Autodesk Inventor part; units mm, degrees
ref_plane "YZ Plane" through (0, 0, 0) normal (1, 0, 0) x (0, 1, 0)
ref_plane "XZ Plane" through (0, 0, 0) normal (0, 1, 0) x (-1, 0, 0)
ref_plane "XY Plane" through (0, 0, 0) normal (0, 0, 1) x (1, 0, 0)
sketch "Sketch1" plane through (0, 0, 0) normal (0, 0, 1) x (1, 0, 0)
  line L0 (21, -21) -> (-21, -21)
  line L1 (-21, -21) -> (-21, 21)
  line L2 (-21, 21) -> (21, 21)
  line L3 (21, 21) -> (21, -21)
  line L4 (21, -21) -> (-21, 21) construction
  line L5 (-21, -21) -> (21, 21) construction
  point P0 (0, 0)
  dimension "d0" = 42
extrude "Extrusion1" add sketch "Sketch1" along normal blind 48
sketch "Sketch2" plane through (0, 0, 48) normal (0, 0, 1) x (1, 0, 0)
  point P0 (0, 0)
  point P1 (-15.5, 15.5)
  point P2 (-15.5, -15.5)
  point P3 (15.5, -15.5)
  point P4 (15.5, 15.5)
  dimension "d3" = 31
  dimension "d4" = 31
  dimension "d5" = 15.5
  dimension "d6" = 15.5
hole "Hole1" at (-15.5, 15.5, 48) at (-15.5, -15.5, 48) at (15.5, -15.5, 48) at (15.5, 15.5, 48) direction (0, 0, -1) diameter 3 depth 8 tip angle 118
chamfer "Chamfer1" distance 3.5 angle 45 4 edges at (21, 21, 24) (21, -21, 24) (-21, 21, 24) (-21, -21, 24)
sketch "Sketch3" plane through (0, 0, 48) normal (0, 0, 1) x (1, 0, 0)
  circle A0 centre (0, 0) radius 11
  dimension "d17" = 22
extrude "Extrusion2" add sketch "Sketch3" along normal blind 2
sketch "Sketch4" plane through (0, 0, 50) normal (0, 0, 1) x (1, 0, 0)
  circle A0 centre (0, 0) radius 11
  circle A1 centre (0, 0) radius 2.5
  dimension "d20" = 5
extrude "Extrusion3" add sketch "Sketch4" along normal blind 25 contours A1
properties part number "Motor_XY" material "Steel, Alloy"
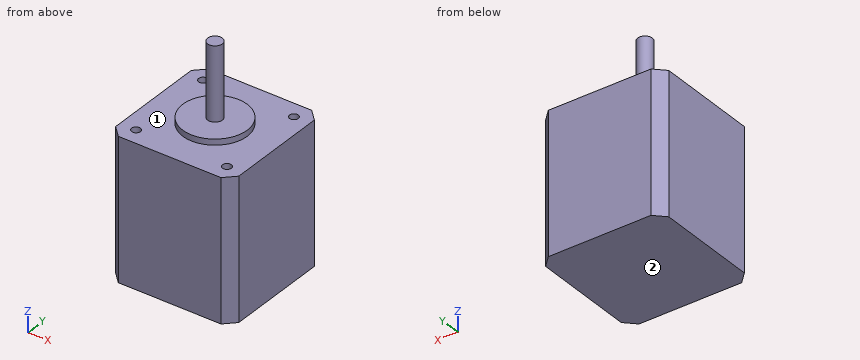
For this review, take the finished solid that the model builds, in its own axes (mm). Face numbers are marked on the shaded views. A direction names the side the tool comes from. Give positions to 0.01 mm unless a question says otherwise; leave off trailing zeros. Loops run counter-clockwise (first coordinate to the right, second up) from the corner with the lowest first, then second, coordinate; pieces in that order, holes last. Notation, with made-up numbers: M 55,62.25 L 108,62.25 A12 ccw 108,83.25 Z; hole C -15,13.25 d5. An arc over 180 degrees is marked long. Put each result on its own line as item: value. Start each with the question number.
(1) For pin 1 (2 mm diameter, centred on x = 7, y = -4, fed in from +Z); pin 2 (3 mm diameter, centred on y = 0.5, z = 56.5, fed in from -X); pin 3 (2.5 mm diameter, centred on x = 15.5, y = -15.5, fed in from +Z), all flat-tipped, find the tip position at first contact; note any pin that passes through.
(2) Wall thickness on L1, parallel to Y at x = 15.5, z = 45.25; L2, parallel to Y at x = -15, z = 46: over which ranges is each line inside the solid? List them lowest first.
(3) Machinability: for the marked faces 1 and 2, which of the approach directions +Z, -Z, +X, -X, +Y, -Y give a long, thin tool a straight path to every point of the face, cutting with its end or side? Answer none if there is none.
(4) Add section D-D, the plane y = 12.5. Write out the cut boundary in (x, z), then the cut area to 3 significant figures.
(5) Add section B-B, the plane x = 6. Write out the cut boundary in (y, z), then the cut area to 3 significant figures.
(6) Add section A-A, the plane y = 0. Write out the cut boundary in (x, z), then the cut area to 4 significant figures.
(7) Add section C-C, the plane z = 62.5. Write out the cut boundary in (x, y).
Result:
1. pin 1: stops at z = 50
1. pin 2: stops at x = -2.5
1. pin 3: stops at z = 39.85
2. L1: y = -21 to -17, -14 to 14, 17 to 21
2. L2: y = -21 to -16.91, -14.09 to 14.09, 16.91 to 21
3. face 1: +Z
3. face 2: -Z, +X, -X, +Y, -Y
4. outline: M -21,0 L 21,0 L 21,48 L -21,48 Z
4. area: 2,020 mm^2
5. outline: M -21,0 L 21,0 L 21,48 L 9.22,48 L 9.22,50 L -9.22,50 L -9.22,48 L -21,48 Z
5. area: 2,050 mm^2
6. outline: M -21,0 L 21,0 L 21,48 L 11,48 L 11,50 L 2.5,50 L 2.5,75 L -2.5,75 L -2.5,50 L -11,50 L -11,48 L -21,48 Z
6. area: 2,185 mm^2
7. outline: C 0,0 d5
